```python
from build123d import *

# Parameters (mm, degrees)
SKETCH_1_R      = 3.25
EXTRUDE_1_DEPTH = 0.8
SKETCH_2_R      = 2.75
EXTRUDE_2_DEPTH = 2.5
CHAMFER_1_SIZE  = 0.8
SKETCH_3_R      = 1
EXTRUDE_3_DEPTH = 0.45
SKETCH_4_W      = 12
SKETCH_4_H      = 12
SKETCH_4_W_2    = 8
SKETCH_4_H_2    = 8
EXTRUDE_4_DEPTH = 0.8


with BuildPart() as part:
    # 草图1 → 凸台-拉伸1 (new body)
    with BuildSketch(Plane(origin=(0, 0, 0), x_dir=(1, 0, 0), z_dir=(0, 1, 0))):
        with Locations((-4.5, 0)):
            Circle(SKETCH_1_R)
        with BuildLine():
            Line((1.33772234, 0.75), (-1.33772234, 0.75))
            ThreePointArc((-1.33772234, 0.75), (-1.272005081, 0.377556356), (-1.25, 0))
            ThreePointArc((-1.25, 0), (-1.272005081, -0.377556356), (-1.33772234, -0.75))
            Line((-1.33772234, -0.75), (1.33772234, -0.75))
            ThreePointArc((1.33772234, -0.75), (1.25, 0), (1.33772234, 0.75))
        make_face()
        with Locations((4.5, 0)):
            Circle(SKETCH_1_R)
    extrude(amount=EXTRUDE_1_DEPTH)

    # 草图2 → 凸台-拉伸2 (add)
    with BuildSketch(Plane(origin=(0, 0.8, 0), x_dir=(1, 0, 0), z_dir=(0, 1, 0))):
        with Locations(Location((-4.5, 0, 0), (0, 0, 270))):
            Circle(SKETCH_2_R)
        with Locations(Location((4.5, 0, 0), (0, 0, 270))):
            Circle(SKETCH_2_R)
    extrude(amount=EXTRUDE_2_DEPTH)

    # 倒角1
    chamfer_1_edges = [part.edges().sort_by_distance(p)[0] for p in [
        (-4.5, 3.3, -2.75),
        (4.5, 3.3, -2.75),
    ]]
    chamfer(chamfer_1_edges, length=CHAMFER_1_SIZE)

    # 草图3 → 凸台-拉伸3 (add)
    with BuildSketch(Plane.XZ):
        with Locations(Location((-4.5, 0, 0), (0, 0, 270))):
            Circle(SKETCH_3_R)
        with Locations(Location((4.5, 0, 0), (0, 0, 90))):
            Circle(SKETCH_3_R)
    extrude(amount=EXTRUDE_3_DEPTH)

    # 草图4 → 凸台-拉伸4 (add)
    with BuildSketch(Plane.XZ):
        with Locations((0, -5)):
            Rectangle(SKETCH_4_W, SKETCH_4_H)
        with Locations((0, -5)):
            Rectangle(SKETCH_4_W_2, SKETCH_4_H_2, mode=Mode.SUBTRACT)
    extrude(amount=-EXTRUDE_4_DEPTH)


solid = part.part
```
Geometry check sheet. Reference: the model listing, model coordinates, mm. A direction names the side the tool comes from. Coordinates: 2 decimals unless noted, no trailing zeros. Write each loop counter-clockwise with the first axis right and the second up, starting at its lowest first coordinate (ties: lowest second). Pieces come first, ordered by that corner, then holes. Notation, with made-up numbers: M 10.25,10.5 L 30.25,10.5 A27 ccw 30.25,27.5 Z; hole C 41.25,28.5 d6. An arc over 180 degrees is marked long. One line per item, written item: value. Start each with the question number.
(1) Release check for a two-part mould opening along X. For faces 1 (the face through (5, 3.3, 0)), 2 (the face through (3.51, -0.22, -0.13)), 3 (the face through (-3.51, -0.22, 0.13)) record: released by +X, released by -X, zero draft, split by the parting line, or undercut.
(2) Depth check by flat-ended pin: pin 1 (2 mm diameter, centred on x = -5.5, y = 2, fed in from +Z); pin 2 (4.5 mm diameter, centred on x = 4, z = -7, fed in from -Y); pin 3 (0.6 mm diameter, centred on x = 2, y = 0.5, fed in from +Z). Enter the tip coordinate at first touch or a pass-through.
(3) Tool access check on faces 4 (the face through (-7.185, 1.638, -0.596)), 5 (the face through (-0.1, 0, -0.6)), 6 (the face through (-2.372, 0.394, -2.456)). Record the directions out of +Z, -Z, +X, -X, +Y, -Y that give a thin tool (end or side, any length) a straight path to the whole face; none if there is none.
(4) Sectioned sample at A-A, the plane z = -3.5. Enter the section's corners in (x, y).
(5) Sectioned sample at D-D, the plane z = 0. Enter the section's corners in (x, y).
(6) Sectioned sample at B-B, the plane x = -4.5. Enter the section's corners in (y, z), and give its area (3 significant figures).
(7) Scan lines: line 1 along X through (y, z) = (1.4, 0); line 2 along X through (y, z) = (0.7, -4.25); line 3 along Z through (x, y) = (-4.5, 0.95). Record each from-to range of solid material in increasing order. Write a range as [from, to].
(8) Sectioned sample at C-C, the plane y = 2.9. Enter the section's corners in (x, z), and give its area (3 significant figures).
Filled sheet:
1. face 1: zero draft
1. face 2: undercut
1. face 3: undercut
2. pin 1: z = 2.75
2. pin 2: y = 0
2. pin 3: z = 2.39
3. face 4: +Y
3. face 5: -Y
3. face 6: +Y, -Y
4. outline: M -6,0 L -4,0 L -4,0.8 L -6,0.8 Z; M 4,0 L 6,0 L 6,0.8 L 4,0.8 Z
5. outline: M -7.75,0 L -5.5,0 L -5.5,-0.45 L -3.5,-0.45 L -3.5,0 L 3.5,0 L 3.5,-0.45 L 5.5,-0.45 L 5.5,0 L 7.75,0 L 7.75,0.8 L 7.25,0.8 L 7.25,2.5 L 6.45,3.3 L 2.55,3.3 L 1.75,2.5 L 1.75,0.8 L -1.75,0.8 L -1.75,2.5 L -2.55,3.3 L -6.45,3.3 L -7.25,2.5 L -7.25,0.8 L -7.75,0.8 Z
6. outline: M -0.45,-1 L 0,-1 L 0,-11 L 0.8,-11 L 0.8,-2.75 L 2.5,-2.75 L 3.3,-1.95 L 3.3,1.95 L 2.5,2.75 L 0.8,2.75 L 0.8,3.25 L 0,3.25 L 0,1 L -0.45,1 Z
6. area: 25.4 mm²
7. line 1: [-7.25, -1.75], [1.75, 7.25]
7. line 2: [-6, -4], [4, 6]
7. line 3: [-2.75, 2.75]
8. outline: C -4.5,0 d4.7; C 4.5,0 d4.7
8. area: 34.7 mm²
